Can you work these out from the model? Positions are in its coordinate system, mm. A direction names the side the tool comes from. Round coordinates to 2 decimals unless told otherwise and drop trailing zeros. Write each loop counter-clockwise with the first axis right and the second up, starting at its lowest first coordinate (ties: lowest second). Pieces come first, ordered by that corner, then holes. Notation, with made-up numbers: (59.25, 59.5) -> (85.25, 59.5) arc R30 cw to (85.25, 88.5) -> close; hole circle Ø3 at (54, 56). An arc over 180 degrees is marked (long way). Write item = value, one per line. Start each with the question number.
1) Imagine slicing it at D-D, the plane x = -7. Please give me the cut outline in (y, z).
2) I'm going to push flat-ended pins straight in: pin 1 (4 mm diameter, centred on x = -1, y = 63.5, fed in from +Z); pin 2 (2 mm diameter, centred on x = 2.5, y = 62, fed in from -Z); pin 3 (3 mm diameter, centred on y = 54, z = -5.5, fed in from -X). Where does each tip first touch, or does it pass through?
3) If I drill on line 1 (X direction, y = 37.5, z = 0); line 2 (X direction, y = 18, z = 0.5); line 3 (Y direction, x = 2.25, z = 6), over which ranges is the centre line in solid material (lowest first)?
4) Imagine slicing it at B-B, the plane y = 120.5. Please give me the cut outline in (x, z) (1 decimal).
5) For faces 1 (the face through (-4, 5.953, 3)), 2 (the face through (0, 145.653, 0)), which set-ups out of +Z, -Z, +X, -X, +Y, -Y let a thin tool reach every point of the face, with its end or its side?
6) Imagine slicing it at C-C, the plane z = 2.25. Please give me the cut outline in (x, y), then the cut area to 3 significant figures.
7) Imagine slicing it at A-A, the plane x = 0. Please give me the cut outline in (y, z).
Autodesk Inventor part; units mm, degrees
ref_plane "YZ Plane" through (0, 0, 0) normal (1, 0, 0) x (0, 1, 0)
ref_plane "XZ Plane" through (0, 0, 0) normal (0, 1, 0) x (-1, 0, 0)
ref_plane "XY Plane" through (0, 0, 0) normal (0, 0, 1) x (1, 0, 0)
sketch "Sketch1" plane through (0, 0, 0) normal (0, 1, 0) x (-1, 0, 0)
  line L0 (-4.1244, -7.1437) -> (-8.2489, 0)
  line L1 (-8.2489, 0) -> (-4.1244, 7.1438)
  line L2 (-4.1244, 7.1438) -> (4.1244, 7.1438)
  line L3 (4.1244, 7.1438) -> (8.2489, 0)
  line L4 (8.2489, 0) -> (4.1244, -7.1437)
  line L5 (4.1244, -7.1437) -> (-4.1244, -7.1437)
  point P0 (0, 0)
  point P1 (0, 0)
  dimension "d0" = 14.2875
extrude "Extrusion1" add sketch "Sketch1" along normal blind 5.9531
sketch "Sketch2" plane through (0, 5.9531, 0) normal (0, 1, 0) x (1, 0, 0)
  circle A0 centre (0, 0) radius 4.7625
  dimension "d3" = 9.525
extrude "Extrusion2" add sketch "Sketch2" along normal blind 139.7
properties part number "half-inch hex bolt" material "Steel, Cast"
Reported:
q1.outline = (0, -2.16) -> (5.95, -2.16) -> (5.95, 2.16) -> (0, 2.16) -> close
q2.pin_1 = 4.76
q2.pin_2 = -4.52
q2.pin_3 = -2.58
q3.line_1 = -4.76 to 4.76
q3.line_2 = -4.74 to 4.74
q3.line_3 = 0 to 5.95
q4.outline = circle Ø9.5 at (0, 0)
q5.face_1 = +Y
q5.face_2 = +Z, -Z, +X, -X, +Y
q6.outline = (-6.95, 0) -> (6.95, 0) -> (6.95, 5.95) -> (4.2, 5.95) -> (4.2, 145.65) -> (-4.2, 145.65) -> (-4.2, 5.95) -> (-6.95, 5.95) -> close
q6.area = 1,260 mm²
q7.outline = (0, -7.14) -> (5.95, -7.14) -> (5.95, -4.76) -> (145.65, -4.76) -> (145.65, 4.76) -> (5.95, 4.76) -> (5.95, 7.14) -> (0, 7.14) -> close
